For this review, take the finished solid that the model builds, in its own axes (mm). Face numbers are marked on the shaded views. A direction names the side the tool comes from. Coordinates: 2 decimals unless noted, no trailing zeros. Write each loop counter-clockwise with the first axis right and the second up, starting at its lowest first coordinate (ties: lowest second). Pieces come first, ordered by that corner, then holes.
1) Insertion check: P1, Ø8, axis at x = -3.5, z = 6, coming from the -Y side; P2, Ø4, axis at x = 8, z = 4.5, coming from the +Y side; P3, Ø2, axis at x = -9, z = 12.5, coming from the +Y side; P4, Ø8, axis at x = 7, y = 2, coming from the -Z side. Each pin has a flat end and moves straight along its axis. Give the tip position at first contact, or say it passes through.
2) For the marked faces 1 and 2, list the 3-axis set-ups (+Z, -Z, +X, -X, +Y, -Y) from which the entire face can be reached by the end or side of a thin tool; tool diameter is ignored.
3) We need section C-C on z = 8. Write out the cut boundary in (x, y).
4) We need section A-A on y = 0. Write out the cut boundary in (x, z), then the cut area to 3 significant figures.
5) To check wall thickness, follow line 1 along X through (y, z) = (0, 6.75); line 2 along Y through (x, z) = (9.5, 5.25); line 3 along Y through (x, z) = (10.75, 17). State the ranges of each line that lie inside material, in increasing order.
from build123d import *

# Parameters (mm, degrees)
F0_R      = 12.5
F1_DEPTH  = 3
F1_FACE_R = 12.5
F2_DEPTH  = 0.5
F2_TAPER  = 45
F3_DEPTH  = 18


with BuildPart() as f1:
    # F0 (on Top) → F1 (new body)
    with BuildSketch(Plane.XY):
        Circle(F0_R)
    extrude(amount=F1_DEPTH)

    # F1_face (on face) → F2 (join)
    with BuildSketch(Plane.XY.offset(3)):
        Circle(F1_FACE_R)
    extrude(amount=F2_DEPTH, taper=F2_TAPER)

    # F3 (add): a face of the model
    f3_faces = [f1.faces().sort_by_distance(p)[0] for p in [
        (0, 0, 3.5),
    ]]
    extrude(f3_faces, amount=F3_DEPTH)


solid = f1.part
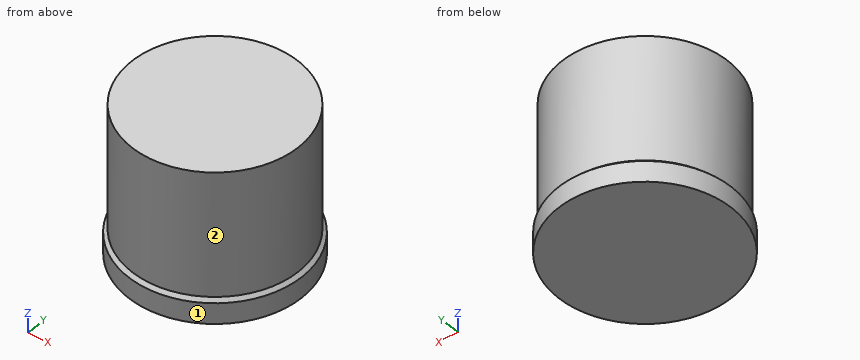
Result:
1. P1: stops at y = -12.47
1. P2: stops at y = 10.57
1. P3: stops at y = 8.94
1. P4: stops at z = 0
2. face 1: +Z, -Z
2. face 2: +Z
3. outline: circle Ø24 at (0, 0)
4. outline: (-12.5, 0) - (12.5, 0) - (12.5, 3) - (12, 3.5) - (12, 21.5) - (-12, 21.5) - (-12, 3.5) - (-12.5, 3) - close
4. area: 519 mm2
5. line 1: x = -12 to 12
5. line 2: y = -7.33 to 7.33
5. line 3: y = -5.33 to 5.33
